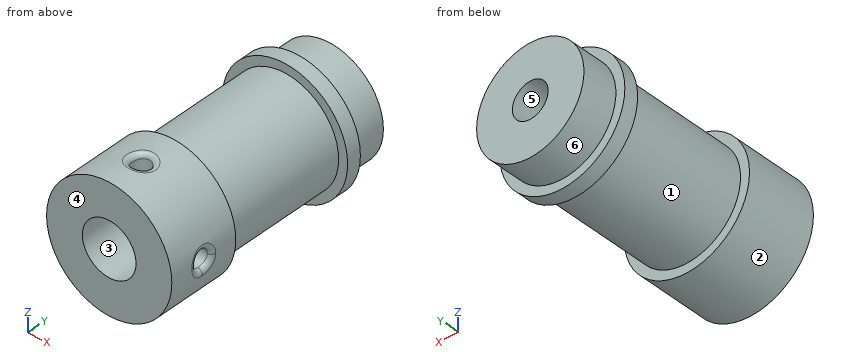
```python
from build123d import *

# Parameters (mm, degrees)
SKETCH1_R           = 7
BOSS_EXTRUDE1_DEPTH = 8
SKETCH2_R           = 6
BOSS_EXTRUDE2_DEPTH = 14
SKETCH3_R           = 7
BOSS_EXTRUDE3_DEPTH = 1.6
SKETCH4_R           = 6
BOSS_EXTRUDE4_DEPTH = 4
SKETCH5_R           = 2
CUT_EXTRUDE1_DEPTH  = 28.6
SKETCH6_R           = 3
CUT_EXTRUDE2_DEPTH  = 20
CUT_EXTRUDE3_START  = -4.171573
SKETCH8_R           = 1
CUT_EXTRUDE3_DEPTH  = 4.171573
CIRPATTERN1_COUNT   = 2
CIRPATTERN1_ANGLE   = 90
FILLET1_R           = 0.5


with BuildPart() as part:
    # Sketch1 → Boss-Extrude1 (new body)
    with BuildSketch(Plane(origin=(0, 0, 0), x_dir=(1, 0, 0), z_dir=(0, 1, 0))):
        Circle(SKETCH1_R)
    extrude(amount=BOSS_EXTRUDE1_DEPTH)

    # Sketch2 → Boss-Extrude2 (add)
    with BuildSketch(Plane(origin=(0, 8, 0), x_dir=(1, 0, 0), z_dir=(0, 1, 0))):
        Circle(SKETCH2_R)
    extrude(amount=BOSS_EXTRUDE2_DEPTH)

    # Sketch3 → Boss-Extrude3 (add)
    with BuildSketch(Plane(origin=(0, 22, 0), x_dir=(1, 0, 0), z_dir=(0, 1, 0))):
        Circle(SKETCH3_R)
    extrude(amount=BOSS_EXTRUDE3_DEPTH)

    # Sketch4 → Boss-Extrude4 (add)
    with BuildSketch(Plane(origin=(0, 23.6, 0), x_dir=(1, 0, 0), z_dir=(0, 1, 0))):
        Circle(SKETCH4_R)
    extrude(amount=BOSS_EXTRUDE4_DEPTH)

    # Sketch5 → Cut-Extrude1 (cut, through all)
    with BuildSketch(Plane(origin=(0, 27.6, 0), x_dir=(1, 0, 0), z_dir=(0, 1, 0))):
        Circle(SKETCH5_R)
    extrude(amount=-CUT_EXTRUDE1_DEPTH, mode=Mode.SUBTRACT)

    # Sketch6 → Cut-Extrude2 (cut)
    with BuildSketch(Plane.XZ):
        Circle(SKETCH6_R)
    extrude(amount=-CUT_EXTRUDE2_DEPTH, mode=Mode.SUBTRACT)

    # Sketch8 → Cut-Extrude3 (cut)
    with BuildSketch(Plane.XY.offset(7).offset(CUT_EXTRUDE3_START)):
        with Locations((0, 4)):
            Circle(SKETCH8_R)
    cut_extrude3 = extrude(amount=CUT_EXTRUDE3_DEPTH, mode=Mode.SUBTRACT)

    # CirPattern1: Cut-Extrude3 ×2 about axis
    cirpattern1_axis = Axis((0, 0, 0), (0, 1, 0))
    for i in range(1, CIRPATTERN1_COUNT):
        add(cut_extrude3.rotate(cirpattern1_axis, i * CIRPATTERN1_ANGLE / (CIRPATTERN1_COUNT - 1)), mode=Mode.SUBTRACT)

    # Fillet1
    fillet1_edges = [part.edges().sort_by_distance(p)[0] for p in [
        (-1, 4, 6.92820323),
        (6.92820323, 4, 1),
    ]]
    fillet(fillet1_edges, radius=FILLET1_R)


solid = part.part
```
Part model, mm, in its own coordinate system. Face numbers are marked on the shaded views. A direction names the side the tool comes from. Round coordinates to 2 decimals unless told otherwise and drop trailing zeros. Loops run counter-clockwise (first coordinate to the right, second up) from the corner with the lowest first, then second, coordinate; pieces in that order, holes last. Notation, with made-up numbers: (-8, -13.75) -> (-2, -13.75) arc R26 ccw to (-2, 2.25) -> close; hole circle Ø6 at (25, 67.5). An arc over 180 degrees is marked (long way). Use CSV: the item, a comma, the result in double quotes. Start each with the question number.
1) Wall check: L1, parallel to Z at x = 0, y = 12.5; L2, parallel to Y at x = 0, z = 4.6; L3, parallel to Y at x = -6, z = 1. Give the ranges that are in metal, low to high. Write a range as [from, to].
2) Cut at A-A, the plane x = 4. Write the cut outline in (y, z), plus the area to 3 significant figures.
3) Which spindle directions (+Z, -Z, +X, -X, +Y, -Y) get a long thin tool onto all of the face, cutting with end or side? Do the marked faces 1, 2 and 3. Say none if no direction does.
4) Cut at B-B, the plane y = 23. Write the cut outline in (x, z).
5) Cut at D-D, the plane y = 9.5. Write the cut outline in (x, z), plus the area to 3 significant figures.
6) Cut at C-C, the plane z = -4.5. Write the cut outline in (x, y).
7) Drop flat-ended pins along their axis: P1, Ø2, axis at y = 16, z = 4.5, coming from the -X side; P2, Ø1.5, axis at x = 2, y = 12.5, coming from the +Z side; P3, Ø5.5, axis at x = 0, z = 0, coming from the -Y side. Give the stop position or say it passes through.
8) Pull direction X, two halves, no side cores. Call the marked faces 4, 5 and 6: +X half, -X half, draft (parallel to the pull), parting line (faces both ways), or undercut.
Determined:
1,L1,"z = [-6, -3], [3, 6]"
1,L2,"y = [0, 3], [5, 27.6]"
1,L3,"y = [0, 8], [22, 23.6]"
2,outline,"(0, -5.74) -> (8, -5.74) -> (8, -4.47) -> (22, -4.47) -> (22, -5.74) -> (23.6, -5.74) -> (23.6, -4.47) -> (27.6, -4.47) -> (27.6, 4.47) -> (23.6, 4.47) -> (23.6, 5.74) -> (22, 5.74) -> (22, 4.47) -> (8, 4.47) -> (8, 5.74) -> (0, 5.74) -> close; hole circle Ø2 at (4, 0)"
2,area,"268 mm2"
3,face 1,"none"
3,face 2,"+Y, -Y"
3,face 3,"-Y"
4,outline,"circle Ø14 at (0, 0); hole circle Ø4 at (0, 0)"
5,outline,"circle Ø12 at (0, 0); hole circle Ø6 at (0, 0)"
5,area,"84.8 mm2"
6,outline,"(-5.36, 0) -> (5.36, 0) -> (5.36, 8) -> (3.97, 8) -> (3.97, 22) -> (5.36, 22) -> (5.36, 23.6) -> (3.97, 23.6) -> (3.97, 27.6) -> (-3.97, 27.6) -> (-3.97, 23.6) -> (-5.36, 23.6) -> (-5.36, 22) -> (-3.97, 22) -> (-3.97, 8) -> (-5.36, 8) -> close"
7,P1,"stops at x = -4.87"
7,P2,"stops at z = 5.87"
7,P3,"stops at y = 20"
8,face 4,"draft"
8,face 5,"undercut"
8,face 6,"parting line"
